Check sheet for the modelled part. Datum: model origin and axes. Units: mm. A direction names the side the tool comes from. Coordinates: 2 decimals unless noted, no trailing zeros. Loops run counter-clockwise (first coordinate to the right, second up) from the corner with the lowest first, then second, coordinate; pieces in that order, holes last. Notation, with made-up numbers: M 43.5,29.5 L 84.5,29.5 A18 cw 84.5,48.5 Z; hole C 50,29 d4. An arc over 180 degrees is marked long. Write each question's results on one line, items separated by ' | '. Start each with the question number.
from build123d import *

# Parameters (mm, degrees)
BOSS_EXTRUDE1_DEPTH = 31.75
SKETCH2_R           = 11.25
SKETCH2_R_2         = 4.5
CUT_EXTRUDE1_DEPTH  = 3.5
CUT_EXTRUDE2_REACH  = 68.912
SKETCH3_R           = 4.5
SKETCH4_W           = 5
SKETCH4_H           = 31.75
CUT_EXTRUDE3_DEPTH  = 2
CHAMFER3_SIZE       = 0.25


with BuildPart() as part:
    # Sketch1 → Boss-Extrude1 (new body)
    with BuildSketch(Plane.XY):
        with BuildLine():
            Line((-22.425, -58.353679699), (-22.425, -28.204472455))
            ThreePointArc((-22.425, -28.204472455), (-22.831389341, -27.223361796), (-23.8125, -26.816972455))
            Line((-23.8125, -26.816972455), (-30.425, -26.816972455))
            Line((-30.425, -26.816972455), (-30.425, -58.353679699))
            Line((-30.425, -58.353679699), (-22.425, -58.353679699))
        make_face()
    extrude(amount=-BOSS_EXTRUDE1_DEPTH)

    # Sketch2 → Cut-Extrude1 (cut)
    with BuildSketch(Plane.ZY.offset(30.425)):
        with Locations((-15.875, -42.478679699)):
            Circle(SKETCH2_R)
        with Locations((-15.875, -42.478679699)):
            Circle(SKETCH2_R_2, mode=Mode.SUBTRACT)
    extrude(amount=-CUT_EXTRUDE1_DEPTH, mode=Mode.SUBTRACT)

    # Sketch3 → Cut-Extrude2 (cut, up to next)
    with BuildSketch(Plane.ZY.offset(30.425), mode=Mode.PRIVATE) as cut_extrude2_sk1:
        with Locations((-15.875, -42.478679699)):
            Circle(SKETCH3_R)
    cut_extrude2_tool1 = extrude(cut_extrude2_sk1.sketch, amount=-CUT_EXTRUDE2_REACH, mode=Mode.PRIVATE) & part.part
    add(cut_extrude2_tool1.solids().sort_by_distance((-30.425, -42.47868, -15.875))[0], mode=Mode.SUBTRACT)

    # Sketch4 → Cut-Extrude3 (cut)
    with BuildSketch(Plane.XZ.offset(58.353679699)):
        with Locations((-26.341152568, -15.875)):
            Rectangle(SKETCH4_W, SKETCH4_H)
    extrude(amount=-CUT_EXTRUDE3_DEPTH, mode=Mode.SUBTRACT)

    # Chamfer3
    chamfer3_edges = [part.edges().sort_by_distance(p)[0] for p in [
        (-30.425, -42.478679699, -27.125),
    ]]
    chamfer(chamfer3_edges, length=CHAMFER3_SIZE)


solid = part.part
Item 1: Depth check by flat-ended pin: P1, Ø4, axis at x = -27.5, z = -17, coming from the -Y side; P2, Ø14.5, axis at y = -42.48, z = -15.88, coming from the -X side (3 decimals). Enter the tip coordinate at first touch or a pass-through.
Item 2: Thickness scan on line 1 (X direction, y = -32.5, z = -19) (3 decimals); line 2 (Z direction, x = -26.5, y = -43.5); line 3 (Y direction, x = -25.75, z = -10). Record the ranges inside material, lowest first.
Item 3: Tool access check on faces 5 (the face through (-23.841, -57, -16)), 6 (the face through (-26.925, -42, -11)), 7 (the face through (-22.821, -27.234, -15.653)). Record the directions out of +Z, -Z, +X, -X, +Y, -Y that give a thin tool (end or side, any length) a straight path to the whole face; none if there is none.
Item 4: Section check C-C (x = -23). Record the cut outline in (y, z) (3 decimals).
Item 5: Section check A-A (z = -28). Record the cut outline in (x, y) (1 decimal), plus the area to 3 significant figures.
Item 6: Release check for a two-part mould opening along X. For faces 1 (the face through (-26, -56.354, -16)), 2 (the face through (-30.425, -32, -9)), 3 (the face through (-28.841, -57, -16)), 4 (the face through (-24.706, -38.017, -16.461)) record: +X half, -X half, draft (parallel to the pull), parting line (faces both ways), or undercut.
Item 7: Section check B-B (x = -29.25). Record the cut outline in (y, z) (3 decimals).
Computed values:
1) P1: stops at y = -58.35 | P2: stops at x = -26.925
2) line 1: x = -26.925 to -22.425 | line 2: z = -31.75 to -20.26, -11.49 to 0 | line 3: y = -56.35 to -26.82
3) face 5: +Z, -Z, -Y | face 6: -X | face 7: +Z, -Z, +X, +Y
4) outline: M -58.354,-31.75 L -27.08,-31.75 L -27.08,0 L -58.354,0 Z; hole C -42.479,-15.875 d9
5) outline: M -30.4,-58.4 L -28.8,-58.4 L -28.8,-56.4 L -23.8,-56.4 L -23.8,-58.4 L -22.4,-58.4 L -22.4,-28.2 A1.4 ccw -23.8,-26.8 L -30.4,-26.8 Z | area: 242 mm²
6) face 1: undercut | face 2: -X half | face 3: undercut | face 4: draft
7) outline: M -58.354,-31.75 L -26.817,-31.75 L -26.817,0 L -58.354,0 Z; hole C -42.479,-15.875 d22.5
